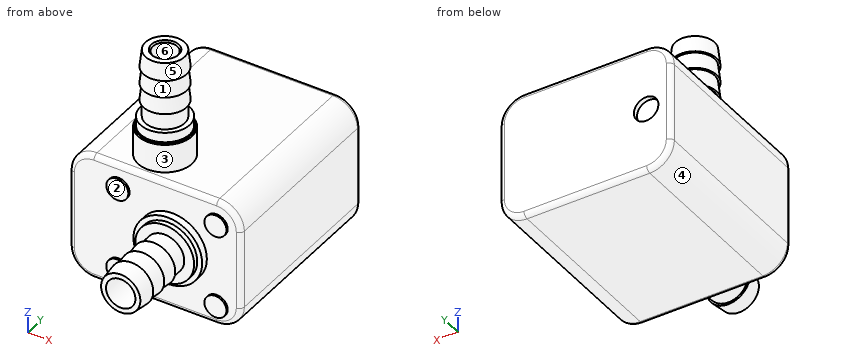
from build123d import *

# Parameters (mm, degrees)
F0_W      = 35
F0_H      = 38
F1_DEPTH  = 26
F2_R      = 5.5
F2_R_2    = 2.75
F3_DEPTH  = 6
F4_R      = 5
F4_R_2    = 2.75
F5_DEPTH  = 2
F9_SIZE   = 0.3
F10_SIZE  = 0.2
F11_R     = 5
F12_R     = 1
F13_R     = 7
F13_R_2   = 3
F14_DEPTH = 1.5
F15_R     = 6
F15_R_2   = 3
F16_DEPTH = 1
F20_R     = 2.25
F21_DEPTH = 0.4
F22_R     = 2.5
F23_DEPTH = 1


with BuildPart() as f1:
    # F0 (on Top) → F1 (new body)
    with BuildSketch(Plane.XY):
        Rectangle(F0_W, F0_H)
    extrude(amount=F1_DEPTH)

    # F2 (on face) → F3 (join)
    with BuildSketch(Plane.XY.offset(26)):
        with Locations((-2.5, -12)):
            Circle(F2_R)
        with Locations((-2.5, -12)):
            Circle(F2_R_2, mode=Mode.SUBTRACT)
    extrude(amount=F3_DEPTH)

    # F4 (on face) → F5 (join)
    with BuildSketch(Plane.XY.offset(32)):
        with Locations((-2.5, -12)):
            Circle(F4_R)
        with Locations((-2.5, -12)):
            Circle(F4_R_2, mode=Mode.SUBTRACT)
    extrude(amount=F5_DEPTH)

    # F7 (on offset) → F8 (revolve)
    with BuildSketch(Plane.XZ.offset(12)):
        Polygon((-6.5000001341, 37.5), (-6.5000001341, 34), (-5.0000001341, 34), (-5.0000001341, 48), (-6.5000001341, 48), (-6.9000001341, 44.5), (-6.5000001341, 44.5), (-6.9000001341, 41), (-6.5000001341, 41), (-6.9000001341, 37.5), align=None)
    revolve(axis=Axis((-2.5, -12, 43.5864264173), (0, 0, 1)))

    # F9
    f9_edges = [f1.edges().sort_by_distance(p)[0] for p in [
        (0, -12, 48),
    ]]
    chamfer(f9_edges, length=F9_SIZE)

    # F10
    f10_edges = [f1.edges().sort_by_distance(p)[0] for p in [
        (-8, -12, 32),
    ]]
    chamfer(f10_edges, length=F10_SIZE)

    # F11
    f11_edges = [f1.edges().sort_by_distance(p)[0] for p in [
        (-17.5, 0, 26),
        (-17.5, 0, 0),
        (17.5, 0, 26),
        (17.5, 0, 0),
    ]]
    fillet(f11_edges, radius=F11_R)

    # F12
    f12_edges = [f1.edges().sort_by_distance(p)[0] for p in [
        (0, 19, 26),
        (0, -19, 26),
    ]]
    fillet(f12_edges, radius=F12_R)

    # F13 (on face) → F14 (join)
    with BuildSketch(Plane.XZ.offset(19)):
        with Locations((3.5, 13)):
            Circle(F13_R)
        with Locations((3.5, 13)):
            Circle(F13_R_2, mode=Mode.SUBTRACT)
    extrude(amount=F14_DEPTH)

    # F15 (on face) → F16 (join)
    with BuildSketch(Plane.XZ.offset(20.5)):
        with Locations((3.5, 13)):
            Circle(F15_R)
        with Locations((3.5, 13)):
            Circle(F15_R_2, mode=Mode.SUBTRACT)
    extrude(amount=F16_DEPTH)

    # F18 (on offset) → F19 (revolve)
    with BuildSketch(Plane.XY.offset(13)):
        Polygon((0.5, -35.5), (0.5, -21.5), (-0.5, -21.5), (-0.5, -25), (-0.9, -25), (-0.5, -28.5), (-0.9, -28.5), (-0.5, -32), (-0.9, -32), (-0.5, -35.5), align=None)
    revolve(axis=Axis((3.5, -28.1351610951, 13), (0, -1, 0)))

    # F20 (on face) → F21 (join)
    with BuildSketch(Plane.XZ.offset(19)):
        with Locations((-7.5, 21)):
            Circle(F20_R)
        with Locations((12.5, 21)):
            Circle(F20_R)
        with Locations((-7.5, 4)):
            Circle(F20_R)
        with Locations((12.5, 4)):
            Circle(F20_R)
    extrude(amount=F21_DEPTH)

    # F22 (on face) → F23 (cut)
    with BuildSketch(Plane(origin=(0, 19, 0), x_dir=(-1, 0, 0), z_dir=(0, 1, 0))):
        with Locations((12.3899085447, 13)):
            Circle(F22_R)
    extrude(amount=-F23_DEPTH, mode=Mode.SUBTRACT)


solid = f1.part
Geometry check sheet. Reference: the model listing, model coordinates, mm. Face numbers are marked on the shaded views. A direction names the side the tool comes from. Give positions to 0.01 mm unless a question says otherwise; leave off trailing zeros. Write each loop counter-clockwise with the first axis right and the second up, starting at its lowest first coordinate (ties: lowest second). Pieces come first, ordered by that corner, then holes. Notation, with made-up numbers: M -23,43 L -17,43 A31 cw -17,73 Z; hole C 51,31.5 d4. An arc over 180 degrees is marked long. Answer as CSV lines item,"result". Start each with the question number.
Q1. Go/stop test with flat-tipped pins: pin 1 (10 mm diameter, centred on x = -11, y = 6, fed in from +Z); pin 2 (3.5 mm diameter, centred on x = 12, z = 4.5, fed in from -Y); pin 3 (6 mm diameter, centred on y = -25.5, z = 5, fed in from -X); pin 4 (3 mm diameter, centred on x = 8.5, y = -29, fed in from -Z). Record where each tip stops, or that it passes through.
Q2. Release check for a two-part mould opening along Y. For the marked faces 4, 5 and 6 record: pulls with the +Y half, pulls with the -Y half, needs draft (parallel to the pull), parting line crosses it, or undercut.
Q3. Material ranges on L1, parallel to Z at x = 3.5, y = -23; L2, parallel to Y at x = -2.5, z = 28.5; L3, parallel to Y at x = 12, z = 19.5, recorded low to high.
Q4. Section check B-B, the plane z = 36.5. Record the cut outline in (x, y), then the cut area to 3 significant figures.
Q5. Section check A-A, the plane y = 7. Record the cut outline in (x, z).
Q6. Tool access check on the marked faces 1, 2 and 3. Record the directions out of +Z, -Z, +X, -X, +Y, -Y that give a thin tool (end or side, any length) a straight path to the whole face; none if there is none.
Geometry says:
1,pin 1,"z = 26"
1,pin 2,"y = -19.4"
1,pin 3,"through"
1,pin 4,"z = 10.41"
2,face 4,"needs draft"
2,face 5,"parting line crosses it"
2,face 6,"undercut"
3,L1,"9 to 10, 16 to 17"
3,L2,"-17.5 to -14.75, -9.25 to -6.5"
3,L3,"-19.4 to 19"
4,outline,"C -2.5,-12 d8; hole C -2.5,-12 d5"
4,area,"30.6 mm^2"
5,outline,"M -17.5,5 A5 ccw -12.5,0 L 12.5,0 A5 ccw 17.5,5 L 17.5,21 A5 ccw 12.5,26 L -12.5,26 A5 ccw -17.5,21 Z"
6,face 1,"none"
6,face 2,"+Z, -Z, -X, -Y"
6,face 3,"+Z"
